Geometry check sheet. Reference: drawing and pictorial views, mm from the part's lowest x, y, z. Round coordinates to 2 decimals unless told otherwise and drop trailing zeros. Write each loop counter-clockwise with the first axis right and the second up, starting at its lowest first coordinate (ties: lowest second). Pieces come first, ordered by that corner, then holes. Notation, with made-up numbers: M 66,18 L 76,18 A9 cw 76,30 Z; hole C 77,25.5 d4. An arc over 180 degrees is marked long. Answer in a Markdown table with one row per item.
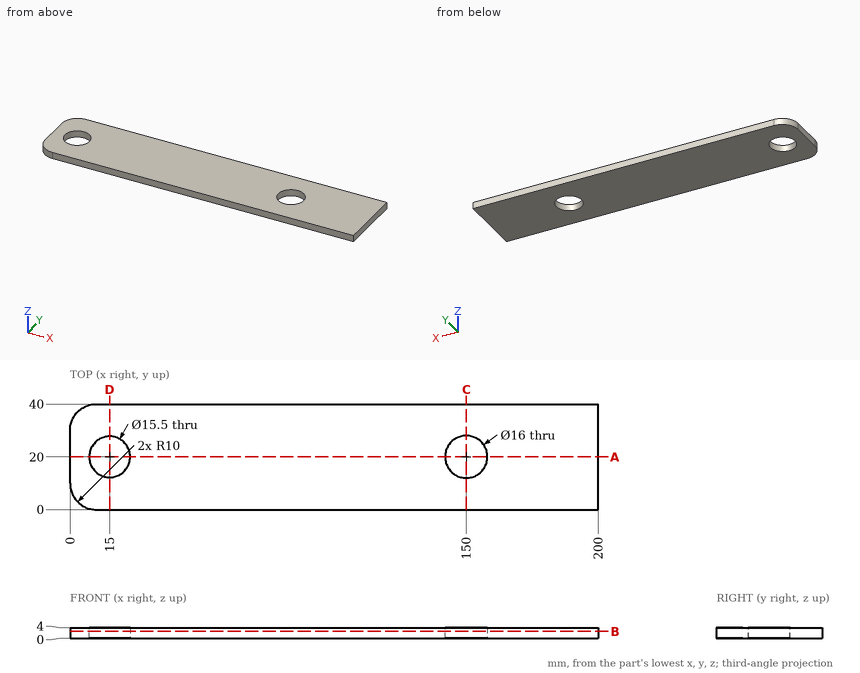
1. Section check C-C, the plane x = 150. Record the cut outline in (y, z).
Found:
| item | result |
|---|---|
| outline | M 0,0 L 12,0 L 12,4 L 0,4 Z; M 28,0 L 40,0 L 40,4 L 28,4 Z |
2. Section check A-A, the plane y = 20. Record the cut outline in (x, z).
Found:
| item | result |
|---|---|
| outline | M 0,0 L 7.25,0 L 7.25,4 L 0,4 Z; M 22.75,0 L 142,0 L 142,4 L 22.75,4 Z; M 158,0 L 200,0 L 200,4 L 158,4 Z |
3. Scan lines: L1, parallel to Y at x = 150, z = 2.15; L2, parallel to Y at x = 15, z = 2; L3, parallel to X at y = 13.5, z = 2.2. Record each from-to range of solid material in increasing order.
Found:
| item | result |
|---|---|
| L1 | y = 0 to 12, 28 to 40 |
| L2 | y = 0 to 12.25, 27.75 to 40 |
| L3 | x = 0 to 10.78, 19.22 to 145.34, 154.66 to 200 |
4. Section check B-B, the plane z = 2.6. Record the cut outline in (x, y), and give its area (3 significant figures).
Found:
| item | result |
|---|---|
| outline | M 0,10 A10 ccw 10,0 L 200,0 L 200,40 L 10,40 A10 ccw 0,30 Z; hole C 15,20 d15.5; hole C 150,20 d16 |
| area | 7,570 mm2 |
5. Section check D-D, the plane x = 15. Record the cut outline in (y, z), and give its area (3 significant figures).
Found:
| item | result |
|---|---|
| outline | M 0,0 L 12.25,0 L 12.25,4 L 0,4 Z; M 27.75,0 L 40,0 L 40,4 L 27.75,4 Z |
| area | 98.0 mm2 |
6. Go/stop test with a flat-tipped pin: pin 1 (9.5 mm diameter, centred on x = 15, y = 20, fed in from +Z). Record where the tip stops, or that it passes through.
Found:
| item | result |
|---|---|
| pin 1 | passes through |
